Geometry check sheet. Reference: drawing and pictorial views, mm from the part's lowest x, y, z. Round coordinates to 2 decimals unless told otherwise and drop trailing zeros. Write each loop counter-clockwise with the first axis right and the second up, starting at its lowest first coordinate (ties: lowest second). Pieces come first, ordered by that corner, then holes.
Item 1: Section check A-A, the plane y = 242. Record the cut outline in (x, z), plus the area to 3 significant figures.
Item 2: Material ranges on line 1 along Z through (x, y) = (4.25, 152.4); line 2 along Y through (x, z) = (1, 105); line 3 along Y through (x, z) = (1.5, 107.95), recorded low to high.
Item 3: Section check D-D, the plane z = 30.5. Record the cut outline in (x, y), plus the area to 3 significant figures.
Item 4: Depth check by flat-ended pin: pin 1 (1.9 mm diameter, centred on x = 2, z = 153, fed in from +Y); pin 2 (1.9 mm diameter, centred on x = 3, y = 260, fed in from -Z) (1 decimal). Enter the tip coordinate at first touch or a pass-through.
Item 5: Section check B-B, the plane x = 5. State how many separate pieces and enclosed holes the cut face has, plus the area to 3 significant figures.
Item 6: Section check C-C, the plane z = 107.95. Record the cut outline in (x, y), plus the area to 3 significant figures.
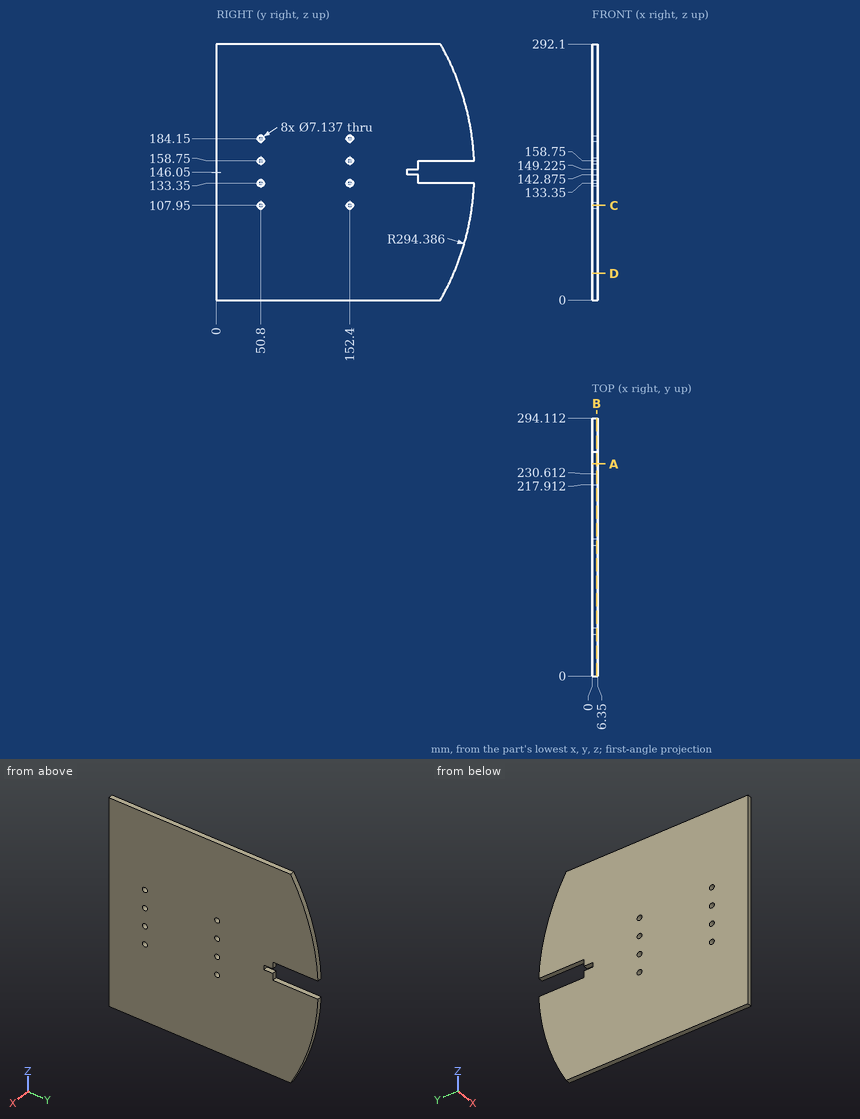
Values found:
1. outline: (0, 0) - (6.35, 0) - (6.35, 133.35) - (0, 133.35) - close; (0, 158.75) - (6.35, 158.75) - (6.35, 292.1) - (0, 292.1) - close
1. area: 1,690 mm2
2. line 1: z = 0 to 104.38, 111.52 to 129.78, 136.92 to 155.18, 162.32 to 180.58, 187.72 to 292.1
2. line 2: y = 0 to 48.79, 52.81 to 150.39, 154.41 to 291.51
2. line 3: y = 0 to 47.23, 54.37 to 148.83, 155.97 to 291.91
3. outline: (0, 0) - (6.35, 0) - (6.35, 270.76) - (0, 270.76) - close
3. area: 1,720 mm2
4. pin 1: stops at y = 230.61
4. pin 2: stops at z = 6.2
5. separate pieces: 1
5. enclosed holes: 8
5. area: 80,300 mm2
6. outline: (0, 0) - (6.35, 0) - (6.35, 47.23) - (0, 47.23) - close; (0, 54.37) - (6.35, 54.37) - (6.35, 148.83) - (0, 148.83) - close; (0, 155.97) - (6.35, 155.97) - (6.35, 291.91) - (0, 291.91) - close
6. area: 1,760 mm2
